The model under review builds one solid part; all positions refer to its coordinate system, in mm. Face numbers are marked on the shaded views. A direction names the side the tool comes from. Give positions to 0.01 mm unless a question says otherwise; leave off trailing zeros. Order: outer loops, then holes, each group sorted by start corner. A loop starts at its lowest first (then second) coordinate and runs counter-clockwise, first axis right, second up. Notation, with made-up numbers: (76, 43) - (108, 43) arc R8 ccw to (108, 50) - close; hole circle Ø4 at (28, 36.5). An arc over 180 degrees is marked (long way). Use CSV: the item, a comma, the result in double quotes. Start each with the question number.
```python
from build123d import *

# Parameters (mm, degrees)
F0_W     = 57.15
F0_H     = 44.45
F1_DEPTH = 25.4
F3_DEPTH = 12.7
F4_DEPTH = 25.4


with BuildPart() as f1:
    # F0 (on Front) → F1 (new body)
    with BuildSketch(Plane.XZ):
        with Locations((28.575, 22.225)):
            Rectangle(F0_W, F0_H)
    extrude(amount=F1_DEPTH)

    # F2 (on face) → F3 (cut)
    with BuildSketch(Plane.XZ.offset(25.4)):
        with BuildLine():
            Line((57.15, 44.45), (19.05, 44.45))
            Line((19.05, 44.45), (22.8288518953, 37.8370091832))
            ThreePointArc((22.8288518953, 37.8370091832), (33.4198634362, 35.2474255755), (38.1, 25.4))
            ThreePointArc((38.1, 25.4), (37.2488826998, 20.8290068075), (34.8096096432, 16.8706831245))
            Line((34.8096096432, 16.8706831245), (44.45, 0))
            Line((44.45, 0), (57.15, 0))
            Line((57.15, 0), (57.15, 44.45))
        make_face()
    extrude(amount=-F3_DEPTH, mode=Mode.SUBTRACT)

    # F2 (on face) → F4 (cut)
    with BuildSketch(Plane.XZ.offset(25.4)):
        with BuildLine():
            Line((34.8096096432, 16.8706831245), (22.8288518953, 37.8370091832))
            ThreePointArc((22.8288518953, 37.8370091832), (14.373312095, 19.0990354829), (34.8096096432, 16.8706831245))
        make_face()
        with BuildLine():
            ThreePointArc((38.1, 25.4), (33.4198634362, 35.2474255755), (22.8288518953, 37.8370091832))
            Line((22.8288518953, 37.8370091832), (34.8096096432, 16.8706831245))
            ThreePointArc((34.8096096432, 16.8706831245), (37.2488826998, 20.8290068075), (38.1, 25.4))
        make_face()
    extrude(amount=-F4_DEPTH, mode=Mode.SUBTRACT)


solid = f1.part
```
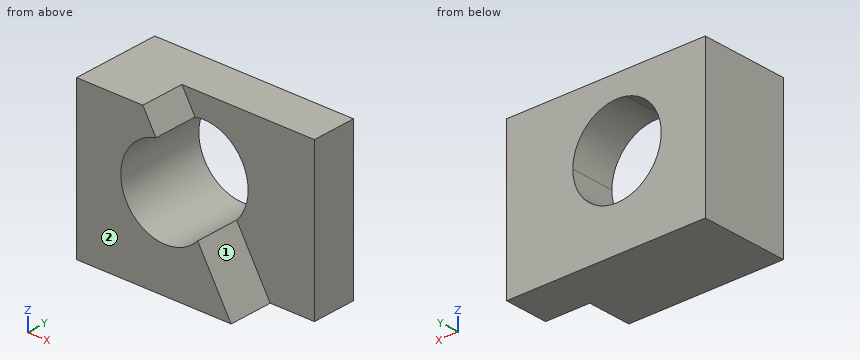
1. To check wall thickness, follow L1, parallel to X at y = -8, z = 25.4; L2, parallel to Y at x = 46, z = 7; L3, parallel to X at y = -14, z = 25.4. State the ranges of each line that lie inside material, in increasing order. Write a range as [from, to].
2. Consider section D-D (y = -17). Give the boundary of the cut face in (x, z).
3. Consider section C-C (y = -7.75). Give the boundary of the cut face in (x, z), and give its area (3 significant figures).
4. Tool access review of the marked faces 1 and 2: name each direction out of +Z, -Z, +X, -X, +Y, -Y from which nothing blocks a thin tool from reaching the whole face with its end or side.
5. Consider section B-B (z = 16). Give the boundary of the cut face in (x, y).
6. Consider section A-A (x = 25.4). Give the boundary of the cut face in (y, z), and give its area (3 significant figures).
7. Clearance check with flat-ended pins moving along their axes: pin 1 (23 mm diameter, centred on x = 25.4, z = 25.4, fed in from +Y); pin 2 (4 mm diameter, centred on y = -11.5, z = 12, fed in from -X); pin 3 (19 mm diameter, centred on x = 42.5, z = 24, fed in from -Y). State where each tip first meets the part, or that it passes through.
Answers follow:
1,L1,"x = [0, 12.7], [38.1, 57.15]"
1,L2,"y = [-12.7, 0]"
1,L3,"x = [0, 12.7]"
2,outline,"(0, 0) - (44.45, 0) - (34.81, 16.87) arc R12.7 cw (long way) to (22.83, 37.84) - (19.05, 44.45) - (0, 44.45) - close"
3,outline,"(0, 0) - (57.15, 0) - (57.15, 44.45) - (0, 44.45) - close; hole circle Ø25.4 at (25.4, 25.4)"
3,area,"2,030 mm^2"
4,face 1,"+Z, +X, -Y"
4,face 2,"+Z, -Z, +X, -X, -Y"
5,outline,"(0, -25.4) - (16.86, -25.4) - (16.86, 0) - (0, 0) - close; (33.94, -25.4) - (35.31, -25.4) - (35.31, -12.7) - (57.15, -12.7) - (57.15, 0) - (33.94, 0) - close"
6,outline,"(-25.4, 0) - (0, 0) - (0, 12.7) - (-25.4, 12.7) - close; (-12.7, 38.1) - (0, 38.1) - (0, 44.45) - (-12.7, 44.45) - close"
6,area,"403 mm^2"
7,pin 1,"passes through"
7,pin 2,"stops at x = 0"
7,pin 3,"stops at y = -12.7"
